Can you work these out from the drawing? Everything is in mm from the part's minimum corner. Round coordinates to 2 decimals unless told otherwise and drop trailing zeros. Loops run counter-clockwise (first coordinate to the right, second up) from the corner with the lowest first, then second, coordinate; pieces in that order, holes last. Notation, with made-up numbers: (51.25, 63.5) -> (89.25, 63.5) arc R12 cw to (89.25, 70.5) -> close; hole circle Ø2 at (13, -38). An arc over 180 degrees is marked (long way). One line per item, written item: value.
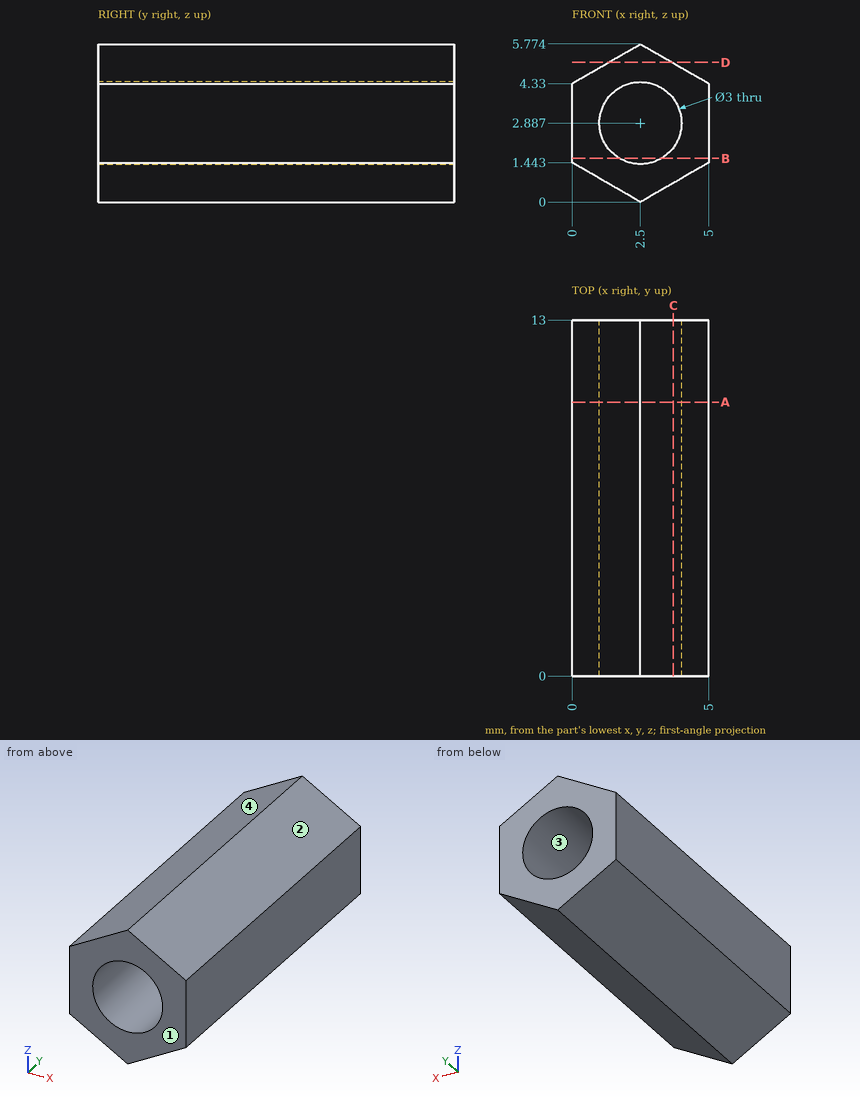
(1) We'd pull the mould along X, two halves only. Please class the marked faces 1, 2, 3 and 4: +X half, -X half, draft (parallel to the pull), parting line (faces both ways), or undercut.
Results below:
face 1: draft
face 2: +X half
face 3: undercut
face 4: -X half
(2) Imagine slicing it at D-D on z = 5.1. Write out the boundary of the cut face in (x, y).
Results below:
outline: (1.33, 0) -> (3.67, 0) -> (3.67, 13) -> (1.33, 13) -> close
(3) Imagine slicing it at A-A on y = 10. Write out the boundary of the cut face in (x, z).
Results below:
outline: (0, 1.44) -> (2.5, 0) -> (5, 1.44) -> (5, 4.33) -> (2.5, 5.77) -> (0, 4.33) -> close; hole circle Ø3 at (2.5, 2.89)
(4) For pin 1 Ø3 at (x, y) = (3.5, 4.5) entering from +Z; pin 2 Ø1.5 at (x, z) = (3, 2.5) entering from -Y, each with a flat end and sliding along its axis, tell me the tip position at first contact or that it passes through.
Results below:
pin 1: stops at z = 5.77
pin 2: passes through
(5) Please list where these lines run through material, in increasing order: L1, parallel to X at y = 4, z = 2.85; L2, parallel to Z at x = 1.5, y = 10.75 (1 decimal); L3, parallel to X at y = 3, z = 4 (1 decimal).
Results below:
L1: x = 0 to 1, 4 to 5
L2: z = 0.6 to 1.8, 4 to 5.2
L3: x = 0 to 1.5, 3.5 to 5
(6) Imagine slicing it at B-B on z = 1.6. Write out the boundary of the cut face in (x, y).
Results below:
outline: (0, 0) -> (1.73, 0) -> (1.73, 13) -> (0, 13) -> close; (3.27, 0) -> (5, 0) -> (5, 13) -> (3.27, 13) -> close
(7) Imagine slicing it at C-C on x = 3.7. Write out the boundary of the cut face in (y, z).
Results below:
outline: (0, 0.69) -> (13, 0.69) -> (13, 1.99) -> (0, 1.99) -> close; (0, 3.79) -> (13, 3.79) -> (13, 5.08) -> (0, 5.08) -> close
